Source: CAD feature listing. Evaluate the final solid. Frame: model axes, mm. A direction names the side the tool comes from. Coordinates: 2 decimals unless noted, no trailing zeros. Loops run counter-clockwise (first coordinate to the right, second up) from the corner with the lowest first, then second, coordinate; pieces in that order, holes last. Notation, with made-up numbers: M 23.5,61.25 L 30.5,61.25 A21 cw 30.5,70.25 Z; hole C -16.75,73.25 d2. An arc over 180 degrees is marked long. Write each question's results on one line, items separated by ' | '. Start each with the question number.
Autodesk Inventor part; units mm, degrees
ref_plane "YZ Plane" through (0, 0, 0) normal (1, 0, 0) x (0, 1, 0)
ref_plane "XZ Plane" through (0, 0, 0) normal (0, 1, 0) x (-1, 0, 0)
ref_plane "XY Plane" through (0, 0, 0) normal (0, 0, 1) x (1, 0, 0)
sketch "Skizze1" plane through (0, 0, 0) normal (0, 1, 0) x (-1, 0, 0)
  line L0 (625.4144, 33.4967) -> (-184.5856, 33.4967)
  line L1 (-184.5856, 33.4967) -> (-184.5856, -108.5033)
  line L2 (-184.5856, -108.5033) -> (625.4144, -108.5033)
  line L3 (625.4144, -108.5033) -> (625.4144, 33.4967)
  line L4 (525.4144, -10.5033) -> (375.4144, -10.5033)
  line L5 (375.4144, -10.5033) -> (375.4144, -64.5033)
  line L6 (375.4144, -64.5033) -> (525.4144, -64.5033)
  line L7 (525.4144, -64.5033) -> (525.4144, -10.5033)
  line L8 (65.4144, -10.5033) -> (-84.5856, -10.5033)
  line L9 (-84.5856, -10.5033) -> (-84.5856, -64.5033)
  line L10 (-84.5856, -64.5033) -> (65.4144, -64.5033)
  line L11 (65.4144, -64.5033) -> (65.4144, -10.5033)
  circle A0 centre (255.4164, -2.5013) radius 3.1
  circle A1 centre (185.3764, -2.5013) radius 3.1
  circle A2 centre (255.4164, -72.5053) radius 3.1
  circle A3 centre (185.3764, -72.5053) radius 3.1
  point P0 (0, 0)
  dimension "d0" = 142
  dimension "d1" = 810
  dimension "d2" = 54
  dimension "d3" = 54
  dimension "d4" = 150
  dimension "d5" = 150
  dimension "d6" = 44
  dimension "d7" = 44
  dimension "d8" = 100
  dimension "d9" = 100
  dimension "d10" = 6.2
  dimension "d11" = 6.2
  dimension "d12" = 6.2
  dimension "d13" = 6.2
  dimension "d14" = 70.004
  dimension "d15" = 0
  dimension "d16" = 0
  dimension "d17" = 70.04
  dimension "d18" = 0
  dimension "d19" = 0
  dimension "d20" = 35.998
  dimension "d21" = 369.998
extrude "Extrusion1" add sketch "Skizze1" against normal blind 20
fillet "Rundung1" radius 2 4 edges at (-220.4144, -20, 33.4967) (-220.4144, 0, 33.4967) (-220.4144, -20, -108.5033) (-220.4144, 0, -108.5033)
properties part number "VerstaerkungHintenMitte"
Item 1: Mould query, pull axis X, two halves, no side actions, for faces 1 (the flat face through (11, -10, -64.503)), 2 (the flat face through (-625.414, -10, -38)), 3 (the flat face through (-215, -20, -37)). Classes: +X half, -X half, draft (parallel to the pull), parting line (faces both ways), or undercut.
Item 2: Cut plane C-C (y = -8.5). Output: boundary loops of the cut face in (x, z), then the cut area to 3 significant figures.
Item 3: Cut plane A-A (x = -16). Output: boundary loops of the cut face in (y, z).
Item 4: Cut plane B-B (z = -19). Output: boundary loops of the cut face in (x, y), then the cut area to 3 significant figures.
Item 5: Access query for faces 4 (the flat face through (-65.414, -10, -38)), 5 (the flat face through (-215, -10, -108.503)). Directions: +Z, -Z, +X, -X, +Y, -Y. A direction counts if a zero-diameter tool reaches every point of the face in a straight line with its end or side. Return the directions, or none.
Item 6: First-contact query: pin 1 Ø5 at (x, z) = (-185.38, -2.5) entering from -Y. Flat tip, straight axial feed; report the tip coordinate or a pass-through.
Item 7: Line query: probe 1 along X at (y, z) = (-4.5, -51); probe 2 along Z at (x, y) = (-442, -16.5); probe 3 along Z at (x, y) = (-253, -14.5). Output: solid intervals per line, ascending.
Response values:
1) face 1: undercut | face 2: -X half | face 3: draft
2) outline: M -625.41,-108.5 L 184.59,-108.5 L 184.59,33.5 L -625.41,33.5 Z; hole M -525.41,-64.5 L -375.41,-64.5 L -375.41,-10.5 L -525.41,-10.5 Z; hole C -255.42,-72.51 d6.2; hole C -255.42,-2.5 d6.2; hole C -185.38,-72.51 d6.2; hole C -185.38,-2.5 d6.2; hole M -65.41,-64.5 L 84.59,-64.5 L 84.59,-10.5 L -65.41,-10.5 Z | area: 98,700 mm2
3) outline: M -20,-106.5 A2 ccw -18,-108.5 L -2,-108.5 A2 ccw 0,-106.5 L 0,-64.5 L -20,-64.5 Z; M -20,-10.5 L 0,-10.5 L 0,31.5 A2 ccw -2,33.5 L -18,33.5 A2 ccw -20,31.5 Z
4) outline: M -625.41,-20 L -525.41,-20 L -525.41,0 L -625.41,0 Z; M -375.41,-20 L -65.41,-20 L -65.41,0 L -375.41,0 Z; M 84.59,-20 L 184.59,-20 L 184.59,0 L 84.59,0 Z | area: 10,200 mm2
5) face 4: +Y, -Y | face 5: -Z, +X, -X, +Y, -Y
6) pin 1: passes through
7) probe 1: x = -625.41 to -525.41, -375.41 to -65.41, 84.59 to 184.59 | probe 2: z = -108.5 to -64.5, -10.5 to 33.5 | probe 3: z = -108.5 to -74.45, -70.56 to -4.44, -0.56 to 33.5
